from build123d import *

# Parameters (mm, degrees)
BOX_W           = 34
BOX_H           = 17
BOX_DEPTH       = 2
SKETCH_R        = 3.25
POCKET_DEPTH    = 2
SKETCH001_W     = 6.498788
SKETCH001_H     = 3.187234
POCKET001_DEPTH = 2
POCKET002_DEPTH = 2
SKETCH003_W     = 12
SKETCH003_H     = 2
PAD_DEPTH       = 2
SKETCH004_W     = 12
SKETCH004_H     = 2
PAD001_DEPTH    = 15
SKETCH005_W     = 12
SKETCH005_H     = 2
PAD002_DEPTH    = 20
PAD003_DEPTH    = 2


with BuildPart() as part:
    # Box → Box (new body)
    with BuildSketch(Plane.XY):
        with Locations((17, 8.5)):
            Rectangle(BOX_W, BOX_H)
    extrude(amount=BOX_DEPTH)

    # Sketch → Pocket (cut)
    with BuildSketch(Plane.XY.offset(2)):
        with Locations((9.25, 11.25)):
            Circle(SKETCH_R)
        with Locations((24.75, 11.25)):
            Circle(SKETCH_R)
        with Locations((17, 3.25)):
            Circle(SKETCH_R)
    extrude(amount=-POCKET_DEPTH, mode=Mode.SUBTRACT)

    # Sketch001 → Pocket001 (cut)
    with BuildSketch(Plane.XY.offset(2)):
        with Locations((17, 1.593617)):
            Rectangle(SKETCH001_W, SKETCH001_H)
    extrude(amount=-POCKET001_DEPTH, mode=Mode.SUBTRACT)

    # Sketch002 → Pocket002 (cut)
    with BuildSketch(Plane.XY.offset(2)):
        Polygon((0, 0), (8, 0), (0, 13), align=None)
        Polygon((34, 0), (26, 0), (34, 13), align=None)
    extrude(amount=-POCKET002_DEPTH, mode=Mode.SUBTRACT)

    # Sketch003 → Pad (new body)
    with BuildSketch(Plane.XZ):
        with Locations((17, 1)):
            Rectangle(SKETCH003_W, SKETCH003_H)
    extrude(amount=PAD_DEPTH)

    # Sketch004 → Pad001 (new body)
    with BuildSketch(Plane.XY.offset(2)):
        with Locations((17, -1)):
            Rectangle(SKETCH004_W, SKETCH004_H)
    extrude(amount=PAD001_DEPTH)

    # Sketch005 → Pad002 (new body)
    with BuildSketch(Plane(origin=(0, 0, 0), x_dir=(1, 0, 0), z_dir=(0, 0, -1))):
        with Locations((17, 1)):
            Rectangle(SKETCH005_W, SKETCH005_H)
    extrude(amount=PAD002_DEPTH)

    # Sketch006 → Pad003 (new body)
    with BuildSketch(Plane.XY.offset(2)):
        Polygon((11, 0), (8, 0), (11, -2), align=None)
        Polygon((23, 0), (26, 0), (23, -2), align=None)
    extrude(amount=-PAD003_DEPTH)


solid = part.part
Input: part model. Units: mm. Frame: model coordinates. A direction names the side the tool comes from. Give positions to 0.01 mm unless a question says otherwise; leave off trailing zeros. Loops run counter-clockwise (first coordinate to the right, second up) from the corner with the lowest first, then second, coordinate; pieces in that order, holes last. Notation, with made-up numbers: (-18, 12) -> (39, 12) arc R23 ccw to (39, 38) -> close; hole circle Ø10 at (-1.75, 57). An arc over 180 degrees is marked (long way). Answer as a JSON object with one key per item and string values. Group by question number.
Item 1: Cut plane D-D, the plane y = 9.25. Return the cut outline in (x, z).
Item 2: Reachability of faces 1 (the flat face through (13.751, 2, 1)), 2 (the flat face through (11, -1, -10)), 3 (the flat face through (23, -1, 10)) from +Z, -Z, +X, -X, +Y, -Y: full face, straight path, thin tool, end or side. Return the list, or none.
Item 3: Cut plane A-A, the plane x = 17. Return the cut outline in (y, z).
Item 4: Pull-direction query (Y, two-part tool) for faces 4 (the flat face through (24.5, -1, 1)), 5 (the flat face through (20.249, 2, 1)), 6 (the flat face through (23, -1, -10)); classes: released by +Y, released by -Y, zero draft, split by the parting line, or undercut.
Item 5: Cut plane C-C, the plane x = 6.5. Return the cut outline in (y, z).
Item 6: Pin query (flat end, axial travel): P1, Ø0.6, axis at y = -1.5, z = 12, coming from the +X side; P2, Ø2, axis at x = 18, z = -3.5, coming from the +Y side; P3, Ø8.5, axis at x = 24.75, y = 11.25, coming from the +Z side. Return the tip coordinate at first contact, or that it passes through.
Item 7: Line query: probe 1 along Y at (x, z) = (13, 12.5); probe 2 along Y at (x, z) = (24.75, 1.6); probe 3 along X at (y, z) = (-0.75, 2.5). Output: solid intervals per line, ascending.
Item 8: Cut plane B-B, the plane y = 12.25. Return the cut outline in (x, z), and give its area (3 significant figures).
Checks:
{
 "1": {"outline": "(2.31, 0) -> (6.69, 0) -> (6.69, 2) -> (2.31, 2) -> close; (11.81, 0) -> (22.19, 0) -> (22.19, 2) -> (11.81, 2) -> close; (27.31, 0) -> (31.69, 0) -> (31.69, 2) -> (27.31, 2) -> close"},
 "2": {"face 1": "+Z, -Z", "face 2": "-Z, -X, +Y, -Y", "face 3": "+Z, +X, +Y, -Y"},
 "3": {"outline": "(-2, -20) -> (0, -20) -> (0, 17) -> (-2, 17) -> close; (6.5, 0) -> (17, 0) -> (17, 2) -> (6.5, 2) -> close"},
 "4": {"face 4": "released by -Y", "face 5": "undercut", "face 6": "zero draft"},
 "5": {"outline": "(2.44, 0) -> (9.52, 0) -> (9.52, 2) -> (2.44, 2) -> close; (12.98, 0) -> (17, 0) -> (17, 2) -> (12.98, 2) -> close"},
 "6": {"P1": "stops at x = 23", "P2": "stops at y = 0", "P3": "stops at z = 2"},
 "7": {"probe 1": "y = -2 to 0", "probe 2": "y = -0.83 to 8, 14.5 to 17", "probe 3": "x = 11 to 23"},
 "8": {"outline": "(0.46, 0) -> (6.16, 0) -> (6.16, 2) -> (0.46, 2) -> close; (12.34, 0) -> (21.66, 0) -> (21.66, 2) -> (12.34, 2) -> close; (27.84, 0) -> (33.54, 0) -> (33.54, 2) -> (27.84, 2) -> close", "area": "41.4 mm²"}
}
